Work out the finished part from the listing and answer in its coordinate system (mm). A direction names the side the tool comes from. Round coordinates to 2 decimals unless told otherwise and drop trailing zeros. Write each loop counter-clockwise with the first axis right and the second up, starting at its lowest first coordinate (ties: lowest second). Pieces come first, ordered by that corner, then holes. Notation, with made-up numbers: M 58.5,36 L 79.5,36 A21 cw 79.5,65 Z; hole C 84,28 d6. An arc over 180 degrees is marked long. One line per item, written item: value. Start each with the question number.
Q1. Find section C-C (y = -38.5). Write down the section's boundary in (x, z) (3 decimals).
Q2. A tool of negligible diameter and unlimited length cuts with its end or side. For faces 5 (the flat face through (-149, -38, -6.35)), 6 (the flat face through (23, 0, -123)), 7 (the flat face through (148, -38, -6.35)), from which of +Z, -Z, +X, -X, +Y, -Y can it reach the whole face along a straight path? Write none if from no direction.
Q3. Find section D-D (x = 0). Write down the section's boundary in (y, z) (3 decimals).
Q4. Find section B-B (z = -12). Write down the section's boundary in (x, y).
Q5. Consider probe 1 along X at (y, z) = (-12, -3); probe 2 along X at (y, z) = (-26, -20); probe 3 along X at (y, z) = (-46, -92.5). Determine where each line is inside the solid, lowest interval first.
Q6. Find section A-A (y = -12.7). Write down the section's boundary in (x, z) (3 decimals), and give its area (3 significant figures).
Q7. The mould has two halves that part along Y. Classify faces 1 (the cylindrical face through (139.834, -67.148, -3.219)), 2 (the cylindrical face through (-157.43, -16.35, -3.22)), 3 (the cylindrical face through (2.774, -37.567, -123.795)), 4 (the flat face through (23, -76.2, -123)): released by +Y, released by -Y, zero draft, split by the parting line, or undercut.
Q8. Given pin 1 Ø3 at (x, y) = (120.5, -35.5) entering from -Z; pin 2 Ø11.5 at (x, y) = (148.63, -63.5) entering from +Z; pin 3 Ø8 at (y, z) = (-22.5, -104.5) entering from -X; pin 4 Ø5 at (x, y) = (-53.5, -48) entering from +Z, each flat-ended and moving along its own axis, determine where each tip first touches the part or whether it passes through.
from build123d import *

# Parameters (mm, degrees)
F1_DEPTH = 76.2
F3_D     = 19.05


with BuildPart() as f1:
    # F0 (on Front) → F1 (new body)
    with BuildSketch(Plane.XZ):
        with BuildLine():
            Line((-161.333019, -6.35), (-135.933019, -6.35))
            ThreePointArc((-135.933019, -6.35), (0, -130.175), (135.933019, -6.35))
            Line((135.933019, -6.35), (161.333019, -6.35))
            Line((161.333019, -6.35), (161.333019, 0))
            Line((161.333019, 0), (130.02003, 0))
            ThreePointArc((130.02003, 0), (0, -123.825), (-130.02003, 0))
            Line((-130.02003, 0), (-161.333019, 0))
            Line((-161.333019, 0), (-161.333019, -6.35))
        make_face()
    extrude(amount=F1_DEPTH)

    # F3 (through all)
    with Locations(Plane.XY):
        with Locations((-148.633019, -63.5), (-148.633019, -12.7), (148.633019, -63.5), (148.633019, -12.7)):
            Hole(F3_D / 2)


solid = f1.part
The answers:
1. outline: M -161.333,-6.35 L -135.933,-6.35 A136.525 ccw 135.933,-6.35 L 161.333,-6.35 L 161.333,0 L 130.02,0 A130.175 cw -130.02,0 L -161.333,0 Z
2. face 5: -Z, -X, +Y, -Y
2. face 6: +Z, -Z, +X, -X, +Y
2. face 7: -Z, +X, +Y, -Y
3. outline: M -76.2,-130.175 L 0,-130.175 L 0,-123.825 L -76.2,-123.825 Z
4. outline: M -135.29,-76.2 L -128.88,-76.2 L -128.88,0 L -135.29,0 Z; M 128.88,-76.2 L 135.29,-76.2 L 135.29,0 L 128.88,0 Z
5. probe 1: -161.33 to -158.13, -139.13 to -129.84, 129.84 to 139.13, 158.13 to 161.33
5. probe 2: -133.96 to -127.48, 127.48 to 133.96
5. probe 3: -94.17 to -84.7, 84.7 to 94.17
6. outline: M -161.333,-6.35 L -158.158,-6.35 L -158.158,0 L -161.333,0 Z; M -139.108,-6.35 L -135.933,-6.35 A136.525 ccw 135.933,-6.35 L 139.108,-6.35 L 139.108,0 L 130.02,0 A130.175 cw -130.02,0 L -139.108,0 Z; M 158.158,-6.35 L 161.333,-6.35 L 161.333,0 L 158.158,0 Z
6. area: 2,660 mm2
7. face 1: undercut
7. face 2: undercut
7. face 3: zero draft
7. face 4: released by -Y
8. pin 1: z = -60.57
8. pin 2: through
8. pin 3: x = -84.98
8. pin 4: z = -111.16
